For this review, take the finished solid that the model builds, in its own axes (mm). A direction names the side the tool comes from. Coordinates: 2 decimals unless noted, no trailing zeros. Loops run counter-clockwise (first coordinate to the right, second up) from the corner with the lowest first, then second, coordinate; pieces in that order, holes last.
```python
from build123d import *

# Parameters (mm, degrees)
SKETCH_1_W          = 28.9
SKETCH_1_H          = 20
EXTRUDE_1_DEPTH     = 8
CUT_EXTRUDE_9_REACH = 38.045
SKETCH_2_R          = 1.5
CUT_EXTRUDE_1_DEPTH = 4


with BuildPart() as part:
    # 草图1 → 凸台-拉伸1 (new body)
    with BuildSketch(Plane.XY):
        with Locations((14.45, 10)):
            Rectangle(SKETCH_1_W, SKETCH_1_H)
    extrude(amount=EXTRUDE_1_DEPTH)

    # 草图3 → 切除-拉伸9 (cut, up to next)
    with BuildSketch(Plane(origin=(28.9, 0, 0), x_dir=(0, 0, -1), z_dir=(1, 0, 0)), mode=Mode.PRIVATE) as cut_extrude_9_sk1:
        Polygon((-8, 15), (-6, 15), (-5, 16.732050808), (-4, 15), (-2, 15), (-2, 5), (-4, 5), (-5, 3.267949192), (-6, 5), (-8, 5), align=None)
    cut_extrude_9_tool1 = extrude(cut_extrude_9_sk1.sketch, amount=-CUT_EXTRUDE_9_REACH, mode=Mode.PRIVATE) & part.part
    add(cut_extrude_9_tool1.solids().sort_by_distance((28.9, 10, 5))[0], mode=Mode.SUBTRACT)

    # 草图2 → 切除-拉伸1 (cut)
    with BuildSketch(Plane(origin=(0, 0, 0), x_dir=(-1, 0, 0), z_dir=(0, 0, -1))):
        with Locations((-19.45, 17.5)):
            Circle(SKETCH_2_R)
        with Locations((-9.45, 17.5)):
            Circle(SKETCH_2_R)
        with Locations((-19.45, 2.5)):
            Circle(SKETCH_2_R)
        with Locations((-9.45, 2.5)):
            Circle(SKETCH_2_R)
    extrude(amount=-CUT_EXTRUDE_1_DEPTH, mode=Mode.SUBTRACT)


solid = part.part
```
Q1. Consider section B-B (z = 7). State the section outline as (x, y) points.
Q2. Consider section C-C (x = 6.5). State the section outline as (y, z) points.
Q3. Consider section A-A (z = 3). State the section outline as (x, y) points.
Q4. Wall thickness on probe 1 along Y at (x, z) = (9.45, 2.85); probe 2 along Y at (x, z) = (4, 3.75); probe 3 along Z at (x, y) = (19, 12.5): over which ranges is each line inside the solid? List them lowest first.
Q5. Consider section D-D (y = 17.5). State the section outline as (x, z) points, then the cut area to 3 significant figures.
Q6. For pin 1 Ø3.5 at (x, y) = (19, 2.5) entering from -Z; pin 2 Ø1.5 at (x, y) = (10, 2.5) entering from -Z; pin 3 Ø3 at (x, y) = (17.5, 8) entering from +Z, all flat-tipped, find the tip position at first contact; note any pin that passes through.
Q7. Machinability: for faces 4 (the face through (8.644, 18.765, 1.972)), 5 (the face through (15, 5, 3)), 6 (the face through (14.65, 4.12, 5.49)), which of the approach directions +Z, -Z, +X, -X, +Y, -Y give a long, thin tool a straight path to every point of the face, cutting with its end or side? Answer none if there is none.
Q8. The part is to be moulded in two halves that separate along X. For faces 1 (the face through (14, 3, 8)), 2 (the face through (8.064, 1.925, 1.972)), 3 (the face through (28.9, 10, 1)), say which applies: +X half, -X half, draft (parallel to the pull), parting line (faces both ways), or undercut.
Model answer:
1. outline: (0, 0) - (28.9, 0) - (28.9, 5) - (0, 5) - close; (0, 15) - (28.9, 15) - (28.9, 20) - (0, 20) - close
2. outline: (0, 0) - (20, 0) - (20, 8) - (15, 8) - (15, 6) - (16.73, 5) - (15, 4) - (15, 2) - (5, 2) - (5, 4) - (3.27, 5) - (5, 6) - (5, 8) - (0, 8) - close
3. outline: (0, 0) - (28.9, 0) - (28.9, 5) - (0, 5) - close; (0, 15) - (28.9, 15) - (28.9, 20) - (0, 20) - close; hole circle Ø3 at (9.45, 2.5); hole circle Ø3 at (9.45, 17.5); hole circle Ø3 at (19.45, 2.5); hole circle Ø3 at (19.45, 17.5)
4. probe 1: y = 0 to 1, 4 to 5, 15 to 16, 19 to 20
4. probe 2: y = 0 to 5, 15 to 20
4. probe 3: z = 0 to 2
5. outline: (0, 0) - (7.95, 0) - (7.95, 4) - (10.95, 4) - (10.95, 0) - (17.95, 0) - (17.95, 4) - (20.95, 4) - (20.95, 0) - (28.9, 0) - (28.9, 8) - (0, 8) - close
5. area: 207 mm2
6. pin 1: stops at z = 0
6. pin 2: stops at z = 4
6. pin 3: stops at z = 2
7. face 4: -Z
7. face 5: +Z, +X, -X
7. face 6: +X, -X
8. face 1: draft
8. face 2: undercut
8. face 3: +X half
